Autodesk Inventor part; units mm, degrees
ref_plane "YZ Plane" through (0, 0, 0) normal (1, 0, 0) x (0, 1, 0)
ref_plane "XZ Plane" through (0, 0, 0) normal (0, 1, 0) x (-1, 0, 0)
ref_plane "XY Plane" through (0, 0, 0) normal (0, 0, 1) x (1, 0, 0)
sketch "Sketch1" plane through (0, 0, 0) normal (0, 0, 1) x (1, 0, 0)
  circle A0 centre (0, 0) radius 3.125
  circle A1 centre (0, 0) radius 1.625
  dimension "d0" = 6.25
  dimension "d1" = 3.25
extrude "Extrusion1" add sketch "Sketch1" along normal blind 5
sketch "Sketch2" plane through (0, 0, 5) normal (0, 0, 1) x (1, 0, 0)
  circle A0 centre (0, 0) radius 3.125
  line L0 (0, 3.125) -> (0, 5.125)
  line L1 (-0.25, 3.125) -> (0.25, 3.125)
  line L2 (0.25, 3.125) -> (0.25, 5.125)
  line L3 (0.25, 5.125) -> (-0.25, 5.125)
  line L4 (-0.25, 5.125) -> (-0.25, 3.125)
  line L5 (-0.25, 3.125) -> (0.25, 5.125) construction
  line L6 (0.25, 3.125) -> (-0.25, 5.125) construction
  line L7 (0, 3.125) -> (0, 2.625)
  line L8 (0, 2.625) -> (0.6, 2.625)
  arc A1 (0.6, 2.625) -> (0.25, 4.125) centre (-2.3986, 2.7162) ccw
  line L9 (0, 2.625) -> (-0.6, 2.625)
  arc A2 (-0.25, 4.125) -> (-0.6, 2.625) centre (2.3986, 2.7162) ccw
  point P0 (0, 4.125)
  point P1 (-1, 2.625)
  dimension "d4" = 2
  dimension "d5" = 0.5
  dimension "d6" = 0.5
  dimension "d7" = 0.6
  dimension "d8" = 1.6
  dimension "d10" = 3
  dimension "d18" = 0.6
  dimension "d19" = 3
extrude "Extrusion2" add sketch "Sketch2" against normal blind 5 contours A1 L8 L7 A0 | A0 L1 L2 A1 | A2 L4 L1 A0 | A0 L7 L9 A2 | L1 L4 L3 L0 | L0 L3 L2 L1
ref_plane "Work Plane1" through (0, 4.125, 5) normal (1, 0, 0) x (0, 0, -1)
sketch "Sketch3" plane through (0, 4.125, 5) normal (1, 0, 0) x (0, 0, -1)
  line L0 (5, -4.125) -> (9.15, -4.125)
pattern_circular "Circular Pattern1" count 18 over 360 about axis through (0, 0, 0) along (0, 0, -1) of "Extrusion2"
properties part number "cog_index"
Geometry: final body of the model. Coordinates: model frame, mm. A direction names the side the tool comes from. Round coordinates to 2 decimals unless told otherwise and drop trailing zeros. Order: outer loops, then holes, each group sorted by start corner. A loop starts at its lowest first (then second) coordinate and runs counter-clockwise, first axis right, second up. Notation, with made-up numbers: (5, -40) -> (37, -40) arc R13 ccw to (37, -20) -> close; hole circle Ø8 at (-9, 58). An arc over 180 degrees is marked (long way). Put each result on its own line as item: value. Start each with the question number.
Q1. Reachability of faces 4 (the flat face through (-4.12, -2.09, 2.54)), 5 (the flat face through (1.814, 4.254, 2.535)), 6 (the flat face through (1.345, -4.425, 2.535)) from +Z, -Z, +X, -X, +Y, -Y: full face, straight path, thin tool, end or side. Return the list, or none.
Q2. Section A-A on x = 0. Return the cut outline in (y, z) (3 decimals).
Q3. Line query: probe 1 along Y at (x, z) = (0, 3.05) (3 decimals); probe 2 along X at (y, z) = (-3, 1.95). Output: solid intervals per line, ascending.
Q4. Pull-direction query (X, two-part tool) for faces 1 (the flat face through (4.14, -2.1, 2.54)), 2 (the flat face through (-1.345, 4.425, 2.535)), 3 (the flat face through (-2, 1, 5)); classes: +X half, -X half, draft (parallel to the pull), parting line (faces both ways), or undercut.
Q5. First-contact query: pin 1 (0.5 mm diameter, centred on y = -4.5, z = 1.5, fed in from -X); pin 2 (1 mm diameter, centred on y = 3.5, z = 2, fed in from -X). Flat tips, straight axial feed; report the tip coordinate or a pass-through.
Ans:
1. face 4: +Z, -Z, -X
1. face 5: +Z, -Z
1. face 6: +Z, -Z, -Y
2. outline: (-5.125, 0) -> (-1.625, 0) -> (-1.625, 5) -> (-5.125, 5) -> close; (1.625, 0) -> (5.125, 0) -> (5.125, 5) -> (1.625, 5) -> close
3. probe 1: y = -5.125 to -1.625, 1.625 to 5.125
3. probe 2: x = -2.84 to -1.87, -1.65 to 1.65, 1.87 to 2.84
4. face 1: +X half
4. face 2: undercut
4. face 3: draft
5. pin 1: stops at x = -1.99
5. pin 2: stops at x = -3.49
